Geometry: final body of the model. Coordinates: model frame, mm. A direction names the side the tool comes from. Give positions to 0.01 mm unless a question says otherwise; leave off trailing zeros. Write each loop counter-clockwise with the first axis right and the second up, starting at its lowest first coordinate (ties: lowest second). Pieces come first, ordered by that corner, then holes. Notation, with made-up numbers: (-15.75, 87) -> (-11.75, 87) arc R24 ccw to (-11.75, 125) -> close; hole circle Ø9 at (82, -15). An arc over 180 degrees is marked (long way). Answer in a Markdown table with one row per item. Add a question column.
Item 1: Draft query along Z for faces 5 (the flat face through (0, 68.5, -8)), 6 (the flat face through (0, 60, -15)), 7 (the flat face through (-12, 112, -8.25)). Return one class per face: +Z half, -Z half, draft (parallel to the pull), parting line (faces both ways), or undercut.
Item 2: Section query D-D on x = -54.5. Output: boundary loops of the cut face in (y, z), plus the area to 3 significant figures.
Item 3: Section query C-C on y = 96. Output: boundary loops of the cut face in (x, z).
Item 4: Access query for faces 1 (the flat face through (-87, 29, 4.5)), 2 (the flat face through (-77.072, 34, -4)), 3 (the flat face through (-1, 103, -15)), 4 (the flat face through (-87, 46, 7)). Directions: +Z, -Z, +X, -X, +Y, -Y. A direction counts if a zero-diameter tool reaches every point of the face in a straight line with its end or side. Return the directions, or none.
Item 5: First-contact query: P1, Ø7.5, axis at x = -2.5, y = 100.5, coming from the -Z side; P2, Ø2.5, axis at x = -128, y = 17.5, coming from the -Z side; P3, Ø0.8, axis at x = -87, z = -3.5, coming from the -Y side; P4, Ø8, axis at x = -104, z = -10.5, coming from the +Y side. Flat tips, straight axial feed; report the tip coordinate or a pass-through.
Item 6: Section query A-A on y = 132. Output: boundary loops of the cut face in (x, z), plus the area to 3 significant figures.
Item 7: Material intervals for probe 1 along X at (y, z) = (20, 2.5); probe 2 along X at (y, z) = (16, -105); probe 3 along Y at (x, z) = (-1, -10), sorted ascending. Write a range as from..to.
```python
from build123d import *
from build123d.topology import SkipClean

# Parameters (mm, degrees)
SKETCH1_W                 = 30
SKETCH1_H                 = 30
BOSS_EXTRUDE1_DEPTH       = 80
SKETCH2_R                 = 6
BOSS_EXTRUDE2_DEPTH       = 20
CUT_EXTRUDE1_DEPTH        = 83.764726786
BOSS_EXTRUDE3_DEPTH       = 65
BOSS_EXTRUDE5_DEPTH       = 2
BOSS_EXTRUDE6_DEPTH       = 23
BOSS_EXTRUDE7_DEPTH       = 25
FILLET1_R                 = 2
SKETCH11_R                = 6.055782361
CUT_EXTRUDE2_DEPTH        = 2.125
CUT_EXTRUDE3_DEPTH        = 238.220050797
CUT_EXTRUDE3_DEPTH_BACK   = 238.220050797
SKETCH12_W                = 13.25
SKETCH12_H                = 8.5
FILLET2_R                 = 2
CUT_EXTRUDE4_REACH        = 195.24
SKETCH15_W                = 3.75
SKETCH15_H                = 3.75
FILLET3_R                 = 1
BOSS_EXTRUDE8_REACH       = 229.962
SKETCH16_W                = 20
SKETCH16_H                = 22
FILLET4_R                 = 2
FILLET5_R                 = 2
SKETCH17_W                = 15
SKETCH17_H                = 17
CUT_EXTRUDE5_DEPTH        = 66
CHAMFER1_SIZE             = 7
BOSS_EXTRUDE9_DEPTH       = 30
BOSS_EXTRUDE10_DEPTH      = 7.999995
BOSS_EXTRUDE10_DEPTH_BACK = 8.000005


with BuildPart() as part:
    # Sketch1 → Boss-Extrude1 (new body)
    with BuildSketch(Plane(origin=(0, 0, 0), x_dir=(1, 0, 0), z_dir=(0, 1, 0))):
        Rectangle(SKETCH1_W, SKETCH1_H)
    extrude(amount=BOSS_EXTRUDE1_DEPTH)

    # Sketch2 → Boss-Extrude2 (add)
    with BuildSketch(Plane(origin=(0, 80, 0), x_dir=(1, 0, 0), z_dir=(0, 1, 0))):
        with Locations(Location((9, -9, 0), (0, 0, 270))):
            Circle(SKETCH2_R)
    extrude(amount=BOSS_EXTRUDE2_DEPTH)

    # Sketch3 → Cut-Extrude1 (cut, through all)
    with BuildSketch(Plane(origin=(0, 80, 0), x_dir=(1, 0, 0), z_dir=(0, 1, 0))):
        with BuildLine():
            Line((9, -15), (15, -15))
            Line((15, -15), (15, -9))
            ThreePointArc((15, -9), (13.242640687, -13.242640687), (9, -15))
        make_face()
    extrude(amount=-CUT_EXTRUDE1_DEPTH, mode=Mode.SUBTRACT)

    # Sketch4 → Boss-Extrude3 (add)
    with BuildSketch(Plane(origin=(0, 80, 0), x_dir=(1, 0, 0), z_dir=(0, 1, 0))):
        Polygon((1.25, 11.25), (1.25, 15), (-1.75, 15), (-1.75, 11.25), (-1.75, 1.75), (-11.25, 1.75), (-15, 1.75), (-15, -1.25), (-11.25, -1.25), (1.25, -1.25), align=None)
        Polygon((-8.25, 11.25), (-8.25, 8.25), (-11.25, 8.25), (-15, 8.25), (-15, 11.25), (-11.25, 11.25), (-11.25, 15), (-8.25, 15), align=None)
    extrude(amount=BOSS_EXTRUDE3_DEPTH)

    # Sketch6 → Boss-Extrude5 (add)
    with BuildSketch(Plane.XZ):
        with BuildLine():
            Line((15, -15), (7, -15))
            Line((7, -15), (7, -99.5))
            ThreePointArc((7, -99.5), (2.757359313, -109.742640687), (13, -105.5))
            Line((13, -105.5), (15, -105.5))
            Line((15, -105.5), (15, -15))
        make_face()
    extrude(amount=-BOSS_EXTRUDE5_DEPTH)

    # Sketch7 → Boss-Extrude6 (add)
    with SkipClean():  # the faces are left unmerged after this step: merging them gives an invalid solid
        with BuildSketch(Plane(origin=(0, 2, 0), x_dir=(1, 0, 0), z_dir=(0, 1, 0))):
            with BuildLine():
                Line((9, 111.156854249), (9, 108.964101615))
                ThreePointArc((9, 108.964101615), (7, 101.5), (5, 108.964101615))
                Line((5, 108.964101615), (5, 111.156854249))
                ThreePointArc((5, 111.156854249), (1.086408642, 104.485388128), (7, 99.5))
                Line((7, 99.5), (7, 15))
                Line((7, 15), (15, 15))
                Line((15, 15), (15, 105.5))
                Line((15, 105.5), (13, 105.5))
                ThreePointArc((13, 105.5), (11.898979486, 108.964101615), (9, 111.156854249))
            make_face()
        extrude(amount=BOSS_EXTRUDE6_DEPTH)

    # Sketch9 → Boss-Extrude7 (add)
    with SkipClean():  # the faces are left unmerged after this step: merging them gives an invalid solid
        with BuildSketch(Plane.XZ):
            with BuildLine():
                Line((-15, 15), (-15, 7))
                Line((-15, 7), (-126.175, 7))
                ThreePointArc((-126.175, 7), (-126.252697751, 6.037536458), (-126.48377869, 5.1))
                Line((-126.48377869, 5.1), (-128.797778509, 5.1))
                ThreePointArc((-128.797778509, 5.1), (-136.05, 7), (-128.797778509, 8.9))
                Line((-128.797778509, 8.9), (-126.3, 8.9))
                ThreePointArc((-126.3, 8.9), (-128.491885554, 11.955834237), (-132.050001601, 13.173329766))
                Line((-132.050001601, 13.173329766), (-132.050001601, 15))
                Line((-132.050001601, 15), (-15, 15))
            make_face()
        extrude(amount=-BOSS_EXTRUDE7_DEPTH)

    # Fillet1
    fillet1_edges = [part.edges().sort_by_distance(p)[0] for p in [
        (-126.175, 12.5, 7),
    ]]
    fillet(fillet1_edges, radius=FILLET1_R)

    # Sketch11 → Cut-Extrude2 (cut)
    with SkipClean():  # the faces are left unmerged after this step: merging them gives an invalid solid
        with BuildSketch(Plane.XZ):
            with Locations((-132.175, 7)):
                Circle(SKETCH11_R)
        extrude(amount=-CUT_EXTRUDE2_DEPTH, mode=Mode.SUBTRACT)

    # Sketch12 → Cut-Extrude3 (cut, two sides: drawn at the far end of the back side and taken through both)
    with SkipClean():  # the faces are left unmerged after this step: merging them gives an invalid solid
        with BuildSketch(Plane(origin=(15, 0, 0), x_dir=(0, 0, -1), z_dir=(1, 0, 0)).offset(-CUT_EXTRUDE3_DEPTH_BACK)):
            with Locations((8.375, 72.75)):
                Rectangle(SKETCH12_W, SKETCH12_H)
        extrude(amount=CUT_EXTRUDE3_DEPTH + CUT_EXTRUDE3_DEPTH_BACK, mode=Mode.SUBTRACT)

    # Fillet2
    fillet2_edges = [part.edges().sort_by_distance(p)[0] for p in [
        (1.25, 112.5, 1.25),
    ]]
    fillet(fillet2_edges, radius=FILLET2_R)

    # Sketch15 → Cut-Extrude4 (cut, up to next)
    with BuildSketch(Plane(origin=(0, 80, 0), x_dir=(1, 0, 0), z_dir=(0, 1, 0)), mode=Mode.PRIVATE) as cut_extrude4_sk1:
        with Locations((-13.125, 13.125)):
            Rectangle(SKETCH15_W, SKETCH15_H)
    cut_extrude4_tool1 = extrude(cut_extrude4_sk1.sketch, amount=-CUT_EXTRUDE4_REACH, mode=Mode.PRIVATE) & part.part
    add(cut_extrude4_tool1.solids().sort_by_distance((-13.125, 80, -13.125))[0], mode=Mode.SUBTRACT)

    # Fillet3
    fillet3_edges = [part.edges().sort_by_distance(p)[0] for p in [
        (-11.25, 112.5, -15),
        (-11.25, 112.5, -11.25),
        (-15, 112.5, -11.25),
        (-15, 112.5, 1.25),
        (1.25, 112.5, -15),
    ]]
    fillet(fillet3_edges, radius=FILLET3_R)

    # Boss-Extrude8: up to this face of the body (flat: up to its plane)
    boss_extrude8_end = Plane(part.part.faces().sort_by_distance((0, 68.5, -8.375))[0])
    # Sketch16 → Boss-Extrude8 (add, up to the picked face)
    with BuildSketch(Plane.XZ, mode=Mode.PRIVATE) as boss_extrude8_sk1:
        with Locations((-87.071774981, -4)):
            Rectangle(SKETCH16_W, SKETCH16_H)
    boss_extrude8_tool1 = split(extrude(boss_extrude8_sk1.sketch, amount=-BOSS_EXTRUDE8_REACH, mode=Mode.PRIVATE), bisect_by=boss_extrude8_end, keep=Keep.BOTH, mode=Mode.PRIVATE)
    add(boss_extrude8_tool1.solids().sort_by(Axis((-87.071775, 0, -4), (0, 1, 0)))[0])

    # Fillet4
    fillet4_edges = [part.edges().sort_by_distance(p)[0] for p in [
        (-77.071774981, 12.5, 7),
        (-77.071774981, 34.25, -15),
        (-97.071774981, 34.25, -15),
        (-97.071774981, 12.5, 7),
    ]]
    fillet(fillet4_edges, radius=FILLET4_R)

    # Fillet5
    fillet5_edges = [part.edges().sort_by_distance(p)[0] for p in [
        (-77.071774981, 46.75, 7),
        (-97.071774981, 46.75, 7),
    ]]
    fillet(fillet5_edges, radius=FILLET5_R)

    # Sketch17 → Cut-Extrude5 (cut)
    with SkipClean():  # the faces are left unmerged after this step: merging them gives an invalid solid
        with BuildSketch(Plane.XZ):
            with Locations((-87.071774981, -4)):
                Rectangle(SKETCH17_W, SKETCH17_H)
        extrude(amount=-CUT_EXTRUDE5_DEPTH, mode=Mode.SUBTRACT)

    # Chamfer1
    chamfer1_edges = [part.edges().sort_by_distance(p)[0] for p in [
        (-94.571774981, 66, -4),
        (-87.071774981, 66, 4.5),
        (-79.571774981, 66, -4),
        (-87.071774981, 66, -12.5),
    ]]
    chamfer(chamfer1_edges, length=CHAMFER1_SIZE)

    # Sketch18 → Boss-Extrude9 (add)
    with SkipClean():  # the faces are left unmerged after this step: merging them gives an invalid solid
        with BuildSketch(Plane(origin=(15, 0, 0), x_dir=(0, 0, -1), z_dir=(1, 0, 0))):
            Polygon((15, 51), (15, 41), (25, 51), align=None)
        extrude(amount=-BOSS_EXTRUDE9_DEPTH)

    # Sketch19 → Boss-Extrude10 (add, two sides: drawn at the far end of the back side and taken through both)
    with SkipClean():  # the faces are left unmerged after this step: merging them gives an invalid solid
        with BuildSketch(Plane.ZY.offset(87.071774981).offset(-BOSS_EXTRUDE10_DEPTH_BACK)):
            Polygon((-15, 41), (-15, 51), (-25, 51), align=None)
        extrude(amount=BOSS_EXTRUDE10_DEPTH + BOSS_EXTRUDE10_DEPTH_BACK)


solid = part.part
```
Findings below:
| question | item | result |
|---|---|---|
| 1 | face 5 | draft |
| 1 | face 6 | -Z half |
| 1 | face 7 | undercut |
| 2 | outline | (0, 7) -> (25, 7) -> (25, 15) -> (0, 15) -> close |
| 2 | area | 200 mm^2 |
| 3 | outline | (-15, -10.25) arc R1 ccw to (-14, -11.25) -> (-12.25, -11.25) arc R1 cw to (-11.25, -12.25) -> (-11.25, -14) arc R1 ccw to (-10.25, -15) -> (-8.25, -15) -> (-8.25, -8.25) -> (-15, -8.25) -> close; (-15, -1.75) -> (-1.75, -1.75) -> (-1.75, -15) -> (0.25, -15) arc R1 ccw to (1.25, -14) -> (1.25, -0.75) arc R2 ccw to (-0.75, 1.25) -> (-14, 1.25) arc R1 ccw to (-15, 0.25) -> close; circle Ø12 at (9, 9) |
| 4 | face 1 | -Y |
| 4 | face 2 | -Z, +Y, -Y |
| 4 | face 3 | -Z, +X, -X, +Y |
| 4 | face 4 | +Z, -X, +Y |
| 5 | P1 | stops at z = -15 |
| 5 | P2 | stops at z = 4.46 |
| 5 | P3 | stops at y = 66 |
| 5 | P4 | passes through |
| 6 | outline | (-15, -10.25) arc R1 ccw to (-14, -11.25) -> (-12.25, -11.25) arc R1 cw to (-11.25, -12.25) -> (-11.25, -14) arc R1 ccw to (-10.25, -15) -> (-8.25, -15) -> (-8.25, -8.25) -> (-15, -8.25) -> close; (-15, -1.75) -> (-1.75, -1.75) -> (-1.75, -15) -> (0.25, -15) arc R1 ccw to (1.25, -14) -> (1.25, -0.75) arc R2 ccw to (-0.75, 1.25) -> (-14, 1.25) arc R1 ccw to (-15, 0.25) -> close |
| 6 | area | 118 mm^2 |
| 7 | probe 1 | x = -97.07..-94.57, -79.57..-77.07, -15..15 |
| 7 | probe 2 | x = 1.02..3.03, 10.97..15 |
| 7 | probe 3 | y = 0..68.5, 77..145 |
